```python
from build123d import *

# Parameters (mm, degrees)
SKETCH_1_R      = 10
EXTRUDE_1_DEPTH = 50
CHAMFER_1_SIZE  = 0.5
SKETCH_2_R      = 15
EXTRUDE_2_DEPTH = 10
CHAMFER_2_SIZE  = 0.5
CHAMFER_3_SIZE  = 0.5
SKETCH_3_R      = 12.5
EXTRUDE_3_DEPTH = 30
CHAMFER_4_SIZE  = 0.5
SKETCH_4_R      = 10
EXTRUDE_4_DEPTH = 30
CHAMFER_5_SIZE  = 0.5
SKETCH_5_R      = 7.5
EXTRUDE_5_DEPTH = 30
CHAMFER_6_SIZE  = 0.5


with BuildPart() as part:
    # 草图1 → 凸台-拉伸1 (new body)
    with BuildSketch(Plane(origin=(0, 0, 0), x_dir=(0, 0, -1), z_dir=(1, 0, 0))):
        Circle(SKETCH_1_R)
    extrude(amount=EXTRUDE_1_DEPTH)

    # 倒角1
    chamfer_1_edges = [part.edges().sort_by_distance(p)[0] for p in [
        (0, 0, 10),
    ]]
    chamfer(chamfer_1_edges, length=CHAMFER_1_SIZE)

    # 草图2 → 凸台-拉伸2 (add)
    with BuildSketch(Plane(origin=(50, 0, 0), x_dir=(0, 0, -1), z_dir=(1, 0, 0))):
        Circle(SKETCH_2_R)
    extrude(amount=EXTRUDE_2_DEPTH)

    # 倒角2
    chamfer_2_edges = [part.edges().sort_by_distance(p)[0] for p in [
        (50, 0, 15),
    ]]
    chamfer(chamfer_2_edges, length=CHAMFER_2_SIZE)

    # 倒角3
    chamfer_3_edges = [part.edges().sort_by_distance(p)[0] for p in [
        (60, 0, 15),
    ]]
    chamfer(chamfer_3_edges, length=CHAMFER_3_SIZE)

    # 草图3 → 凸台-拉伸3 (add)
    with BuildSketch(Plane(origin=(60, 0, 0), x_dir=(0, 0, -1), z_dir=(1, 0, 0))):
        Circle(SKETCH_3_R)
    extrude(amount=EXTRUDE_3_DEPTH)

    # 倒角4
    chamfer_4_edges = [part.edges().sort_by_distance(p)[0] for p in [
        (90, 0, 12.5),
    ]]
    chamfer(chamfer_4_edges, length=CHAMFER_4_SIZE)

    # 草图4 → 凸台-拉伸4 (add)
    with BuildSketch(Plane(origin=(90, 0, 0), x_dir=(0, 0, -1), z_dir=(1, 0, 0))):
        Circle(SKETCH_4_R)
    extrude(amount=EXTRUDE_4_DEPTH)

    # 倒角5
    chamfer_5_edges = [part.edges().sort_by_distance(p)[0] for p in [
        (120, 0, 10),
    ]]
    chamfer(chamfer_5_edges, length=CHAMFER_5_SIZE)

    # 草图5 → 凸台-拉伸5 (add)
    with BuildSketch(Plane(origin=(120, 0, 0), x_dir=(0, 0, -1), z_dir=(1, 0, 0))):
        Circle(SKETCH_5_R)
    extrude(amount=EXTRUDE_5_DEPTH)

    # 倒角6
    chamfer_6_edges = [part.edges().sort_by_distance(p)[0] for p in [
        (150, 0, 7.5),
    ]]
    chamfer(chamfer_6_edges, length=CHAMFER_6_SIZE)


solid = part.part
```
Geometry: final body of the model. Coordinates: model frame, mm. A direction names the side the tool comes from. Coordinates: 2 decimals unless noted, no trailing zeros. Order: outer loops, then holes, each group sorted by start corner. A loop starts at its lowest first (then second) coordinate and runs counter-clockwise, first axis right, second up. Notation, with made-up numbers: M 36,88.5 L 68,88.5 A9 cw 68,102.5 Z; hole C 62.5,55 d6. An arc over 180 degrees is marked long. Answer in a Markdown table with one row per item. Add a question column.
Q1. Section query C-C on x = 42. Return the cut outline in (y, z), and give its area (3 significant figures).
Q2. Section query D-D on x = 65. Return the cut outline in (y, z), and give its area (3 significant figures).
Q3. Reachability of faces 1 (the flat face through (60, 7, 11)), 2 (the cylindrical face through (54.937, 0.66, 14.985)), 3 (the flat face through (50, 10, -3)) from +Z, -Z, +X, -X, +Y, -Y: full face, straight path, thin tool, end or side. Return the list, or none.
Q4. Contact query for flat-ended pins moving along their axis: P1, Ø10, axis at x = 75, z = -3, coming from the -Y side; P2, Ø1.5, axis at y = -8, z = 1, coming from the +X side; P3, Ø1.5, axis at x = 24, z = 7, coming from the +Y side; P4, Ø1, axis at x = 48.5, y = -12, coming from the -Z side. Output: stop coordinate, or through.
Q5. Line query: L1, parallel to X at y = 6, z = -6; L2, parallel to X at y = 5.5, z = -8.75; L3, parallel to Y at x = 125, z = -0.5. Output: solid intervals per line, ascending.
Completed:
| question | item | result |
|---|---|---|
| 1 | outline | C 0,0 d20 |
| 1 | area | 314 mm2 |
| 2 | outline | C 0,0 d25 |
| 2 | area | 491 mm2 |
| 3 | face 1 | +X |
| 3 | face 2 | +X, -X |
| 3 | face 3 | -X |
| 4 | P1 | stops at y = -12.5 |
| 4 | P2 | stops at x = 149.69 |
| 4 | P3 | stops at y = 7.81 |
| 4 | P4 | passes through |
| 5 | L1 | x = 0 to 120 |
| 5 | L2 | x = 50 to 90 |
| 5 | L3 | y = -7.48 to 7.48 |
